```python
from build123d import *

# Parameters (mm, degrees)
SKETCH1_W           = 15
SKETCH1_H           = 15
BOSS_EXTRUDE1_DEPTH = 25
CUT_EXTRUDE1_DEPTH  = 20


with BuildPart() as part:
    # Sketch1 → Boss-Extrude1 (new body)
    with BuildSketch(Plane(origin=(0, 0, 0), x_dir=(1, 0, 0), z_dir=(0, 1, 0))):
        with Locations((7.5, 7.5)):
            Rectangle(SKETCH1_W, SKETCH1_H)
    extrude(amount=BOSS_EXTRUDE1_DEPTH)

    # Sketch2 → Cut-Extrude1 (cut)
    with BuildSketch(Plane(origin=(0, 25, 0), x_dir=(1, 0, 0), z_dir=(0, 1, 0))):
        with BuildLine():
            Line((6, 5.5), (9, 5.5))
            ThreePointArc((9, 5.5), (7.5, 10), (6, 5.5))
        make_face()
    extrude(amount=-CUT_EXTRUDE1_DEPTH, mode=Mode.SUBTRACT)


solid = part.part
```
The listing builds one solid part. Answer for the finished solid, in the listing's coordinates (mm). A direction names the side the tool comes from. Give positions to 0.01 mm unless a question says otherwise; leave off trailing zeros. Write each loop counter-clockwise with the first axis right and the second up, starting at its lowest first coordinate (ties: lowest second). Pieces come first, ordered by that corner, then holes. Notation, with made-up numbers: (-29, 37) -> (21, 37) arc R19 cw to (21, 64) -> close; hole circle Ø5 at (-37.75, -36.5). An arc over 180 degrees is marked (long way). Use one line per item in the form item = value.
1) For a pull along Z with two mould halves and no side action, classify faces 3 (the flat face through (7, 5, -8)), 4 (the flat face through (7, 12, 0)), 5 (the flat face through (4, 25, -8)) as +Z half, -Z half, draft (parallel to the pull), parting line (faces both ways), or undercut.
Result:
face_3 = undercut
face_4 = +Z half
face_5 = draft
2) This flat-tipped pin is pushed along its axis until it touches: P1, Ø5, axis at x = 7.5, z = -7.5, coming from the +Y side. Where does it stop, or does it pass through?
Result:
P1 = 25
3) Section A-A on x = 7.5 is taken. Write down the section's boundary in (y, z), plus the area to 3 significant figures.
Result:
outline = (0, -15) -> (25, -15) -> (25, -10) -> (5, -10) -> (5, -5.5) -> (25, -5.5) -> (25, 0) -> (0, 0) -> close
area = 285 mm²
4) A tool of negligible diameter and unlimited length cuts with its end or side. For faces 1 (the flat face through (15, 12, -7)), 2 (the flat face through (7, 15, -5.5)), from which of +Z, -Z, +X, -X, +Y, -Y can it reach the whole face along a straight path? Write none if from no direction.
Result:
face_1 = +Z, -Z, +X, +Y, -Y
face_2 = +Y
5) Section B-B on y = 19.5 is taken. Write down the section's boundary in (x, z).
Result:
outline = (0, -15) -> (15, -15) -> (15, 0) -> (0, 0) -> close; hole (6, -5.5) arc R2.5 ccw (long way) to (9, -5.5) -> close
6) Straight lines are drawn through the part: probe 1 along Z at (x, y) = (7.5, 10.25); probe 2 along X at (y, z) = (7.5, -9.5); probe 3 along X at (y, z) = (13.75, -7.5). For each, find the intervals that lie inside material, in ascending order.
Result:
probe_1 = -15 to -10, -5.5 to 0
probe_2 = 0 to 6, 9 to 15
probe_3 = 0 to 5, 10 to 15
7) Section C-C on z = -7.5 is taken. Write down the section's boundary in (x, y).
Result:
outline = (0, 0) -> (15, 0) -> (15, 25) -> (10, 25) -> (10, 5) -> (5, 5) -> (5, 25) -> (0, 25) -> close
